Check sheet for the modelled part. Datum: model origin and axes. Units: mm. A direction names the side the tool comes from. Give positions to 0.01 mm unless a question says otherwise; leave off trailing zeros. Write each question's results on one line, items separated by ' | '. Start each with the question number.
Item 1: Scan lines: line 1 along Z through (x, y) = (0.4, -6); line 2 along Z through (x, y) = (0, -5.87) (1 decimal); line 3 along Y through (x, z) = (-0.9, -17). Record each from-to range of solid material in increasing order.
Item 2: Access from +Z, -Z, +X, -X, +Y, -Y to the whole of each face (thin tool, end or side, straight path). Record for faces 1 (the face through (-0.035, 6.732, 17.452)), 2 (the face through (2.204, -5.756, -13.818)), 3 (the face through (-1.9, 8, 15)).
Item 3: Cross-section at A-A on x = -0.75. State how many separate pieces and enclosed holes the cut face has, then the cut area to 3 significant figures.
Item 4: Mould release check, pull along Y, two halves, no side actions. Record for faces 4 (the face through (-2.2, -7.63, -14.5)), 5 (the face through (-0.027, 4.367, 16.202)), 6 (the face through (-0.035, -6.424, -19.465)), 7 (the face through (-2.5, 0, -1)): pulls with the +Y half, pulls with the -Y half, needs draft (parallel to the pull), parting line crosses it, or undercut.
Item 5: Gauge pin test, flat ends, axial feed: pin 1 Ø6 at (y, z) = (-5.87, -16.415) entering from +X; pin 2 Ø4.5 at (y, z) = (5.63, 14.56) entering from -X; pin 3 Ø10 at (y, z) = (5, -12) entering from +X; pin 4 Ø1.6 at (y, z) = (5, 16) entering from +X. Record the tip position at first contact, or that the pin passes through.
from build123d import *

# Parameters (mm, degrees)
BOSS_EXTRUDE1_START     = -2.5
BOSS_EXTRUDE1_OUTLINE_R = 2.075
BOSS_EXTRUDE1_DEPTH     = 5
FILLET1_R               = 10
FILLET2_R               = 2
SKETCH6_R               = 2.6
CUT_EXTRUDE3_DEPTH      = 0.6
CUT_EXTRUDE4_START      = -0.6
SKETCH7_R               = 2.6
CUT_EXTRUDE4_DEPTH      = 0.6


# Read off the part's stored shape, not the designer's step: Boss-Extrude1
with BuildPart() as part:
    # Boss-Extrude1 outline → Boss-Extrude1 (new body)
    with BuildSketch(Plane(origin=(0, 0, 0), x_dir=(0, 0, -1), z_dir=(1, 0, 0)).offset(BOSS_EXTRUDE1_START)):
        with BuildLine():
            add(Edge.make_bspline(
                [(-11.467428758, 5.351849738), (-9.981579618, 4.577281332), (-7.160995192, 3.544086065), (-2.770125707, 2.396619441), (1.347799898, 1.288727674), (5.338957915, -0.215867298), (9.160320461, -1.841071211), (12.08438205, -3.026761323), (13.750853903, -3.610645605), (14.156821659, -3.746175483)],
                knots=[0.086388593, 0.086388593, 0.086388593, 0.086388593, 0.25, 0.375, 0.5, 0.625, 0.75, 0.875, 0.915118366, 0.915118366, 0.915118366, 0.915118366], degree=3))
            ThreePointArc((-11.467428758, 5.351849738), (-17.182273296, 7.274593649), (-12.95766118, 2.972379718))
            add(Edge.make_bspline(
                [(-12.95766118, 2.972379718), (-12.493747453, 2.724314548), (-10.717791227, 1.858624399), (-7.52529105, 0.743374894), (-3.440580849, -0.32158746), (0.497631851, -1.383173076), (4.262093967, -2.802436867), (8.066886426, -4.418200775), (11.094789528, -5.649756293), (12.901972126, -6.280277824), (13.366776805, -6.434212154)],
                knots=[0.08026374, 0.08026374, 0.08026374, 0.08026374, 0.125, 0.25, 0.375, 0.5, 0.625, 0.75, 0.875, 0.917835676, 0.917835676, 0.917835676, 0.917835676], degree=3))
            ThreePointArc((13.366776805, -6.434212154), (19.389198985, -6.744151246), (14.156821659, -3.746175483))
        make_face()
        with Locations((16.415, -5.87)):
            Circle(BOSS_EXTRUDE1_OUTLINE_R, mode=Mode.SUBTRACT)
        with Locations((-14.555, 5.629165125)):
            Circle(BOSS_EXTRUDE1_OUTLINE_R, mode=Mode.SUBTRACT)
    extrude(amount=BOSS_EXTRUDE1_DEPTH)

    # Fillet1
    fillet1_edges = [part.edges().sort_by_distance(p)[0] for p in [
        (0, -6.434212154, -13.366776805),
        (0, 5.351849738, 11.467428758),
    ]]
    fillet(fillet1_edges, radius=FILLET1_R)

    # Fillet2
    fillet2_edges = [part.edges().sort_by_distance(p)[0] for p in [
        (0, -3.746175483, -14.156821659),
        (0, 2.972379718, 12.95766118),
    ]]
    fillet(fillet2_edges, radius=FILLET2_R)

    # Sketch6 → Cut-Extrude3 (cut)
    with BuildSketch(Plane(origin=(2.5, 0, 0), x_dir=(0, 0, -1), z_dir=(1, 0, 0))):
        with Locations((-14.555, 5.629165125)):
            Circle(SKETCH6_R)
        with Locations((16.415, -5.87)):
            Circle(SKETCH6_R)
    extrude(amount=-CUT_EXTRUDE3_DEPTH, mode=Mode.SUBTRACT)

    # Sketch7 → Cut-Extrude4 (cut)
    with BuildSketch(Plane.ZY.offset(2.5).offset(CUT_EXTRUDE4_START)):
        with Locations(Location((14.555, 5.629165125, 0), (0, 0, 180))):
            Circle(SKETCH7_R)
        with Locations(Location((-16.415, -5.87, 0), (0, 0, 180))):
            Circle(SKETCH7_R)
    extrude(amount=CUT_EXTRUDE4_DEPTH, mode=Mode.SUBTRACT)


solid = part.part
Answer sheet:
1) line 1: z = -19.51 to -18.49, -14.34 to -11.72 | line 2: z = -19.5 to -18.5, -14.3 to -11.5 | line 3: y = -8.91 to -7.86, -3.88 to -2.83
2) face 1: +X, -X | face 2: +X | face 3: -X
3) separate pieces: 1 | enclosed holes: 2 | area: 113 mm²
4) face 4: undercut | face 5: undercut | face 6: parting line crosses it | face 7: needs draft
5) pin 1: stops at x = 2.5 | pin 2: stops at x = -1.9 | pin 3: passes through | pin 4: stops at x = 1.9
